The figure shows three views and two pictorial views of one solid part (mm, origin at its lowest corner). Answer the questions. Round coordinates to 2 decimals unless told otherwise and drop trailing zeros. Write each loop counter-clockwise with the first axis right and the second up, starting at its lowest first coordinate (ties: lowest second). Pieces come first, ordered by that corner, then holes. Notation, with made-up numbers: M 57,66 L 108,66 A19 ccw 108,82 Z; hole C 15.25,61 d11. An arc over 180 degrees is marked long. One line per item, written item: value. Start each with the question number.
Q1. The mould has two halves that part along Y. Classify the marked faces 1, 2 and 3: released by +Y, released by -Y, zero draft, split by the parting line, or undercut.
Q2. Given pin 1 Ø1 at (x, z) = (100, 29.5) entering from +Y; pin 2 Ø0.6 at (x, z) = (98.5, 24.5) entering from +Y; pin 3 Ø8 at (y, z) = (23.5, 27) entering from +X, each flat-ended and moving along its own axis, determine where each tip first touches the part or whether it passes through.
Q3. Find section B-B (y = 10.5). Write down the section's boundary in (x, z), and give its area (3 significant figures).
Q4. Find section C-C (z = 15). Write down the section's boundary in (x, y), and give its area (3 significant figures).
Q5. Find section D-D (y = 57). Write down the section's boundary in (x, z), and give its area (3 significant figures).
Q6. Consider probe 1 along Y at (x, z) = (16.5, 8); probe 2 along X at (y, z) = (87, 24). Determine where each line is inside the solid, lowest interval first.
Q7. Find section A-A (x = 10.5). Write down the section's boundary in (y, z).
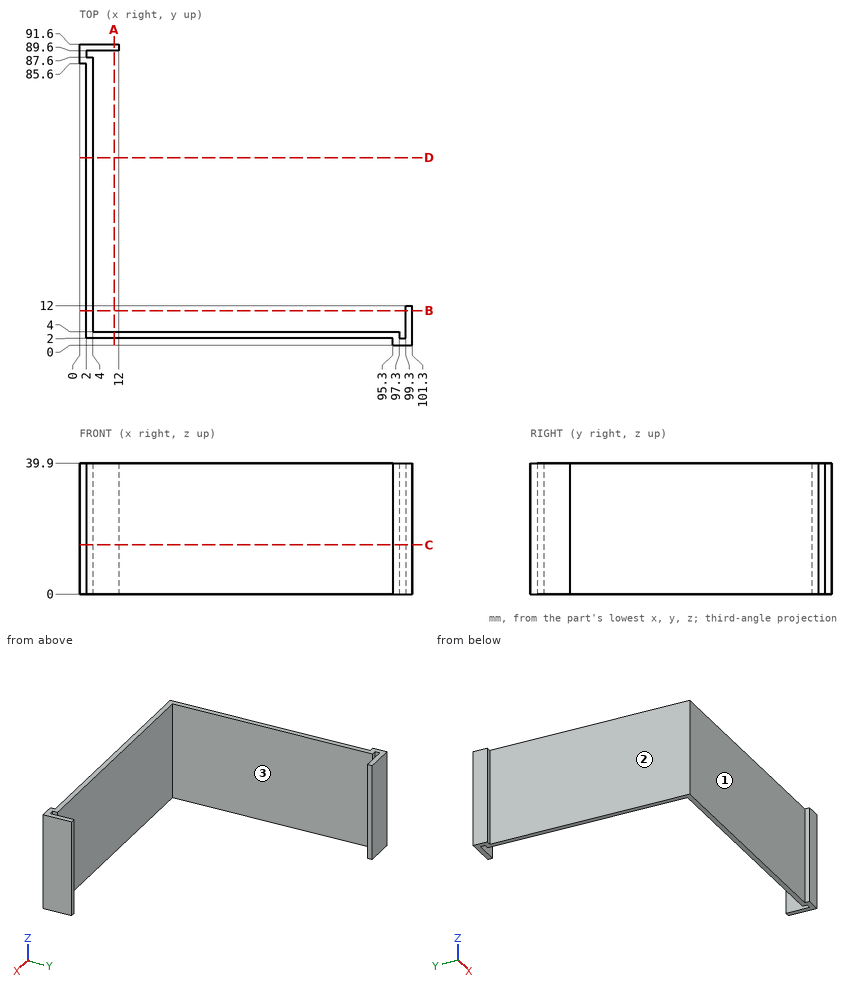
The answers:
1. face 1: released by -Y
1. face 2: zero draft
1. face 3: undercut
2. pin 1: y = 12
2. pin 2: y = 2
2. pin 3: x = 4
3. outline: M 2,0 L 4,0 L 4,39.9 L 2,39.9 Z; M 99.3,0 L 101.3,0 L 101.3,39.9 L 99.3,39.9 Z
3. area: 160 mm2
4. outline: M 0,85.6 L 2,85.6 L 2,2 L 95.3,2 L 95.3,0 L 101.3,0 L 101.3,12 L 99.3,12 L 99.3,2 L 97.3,2 L 97.3,4 L 4,4 L 4,87.6 L 2,87.6 L 2,89.6 L 12,89.6 L 12,91.6 L 0,91.6 Z
4. area: 422 mm2
5. outline: M 2,0 L 4,0 L 4,39.9 L 2,39.9 Z
5. area: 79.8 mm2
6. probe 1: 2 to 4
6. probe 2: 0 to 4
7. outline: M 2,0 L 4,0 L 4,39.9 L 2,39.9 Z; M 89.6,0 L 91.6,0 L 91.6,39.9 L 89.6,39.9 Z
